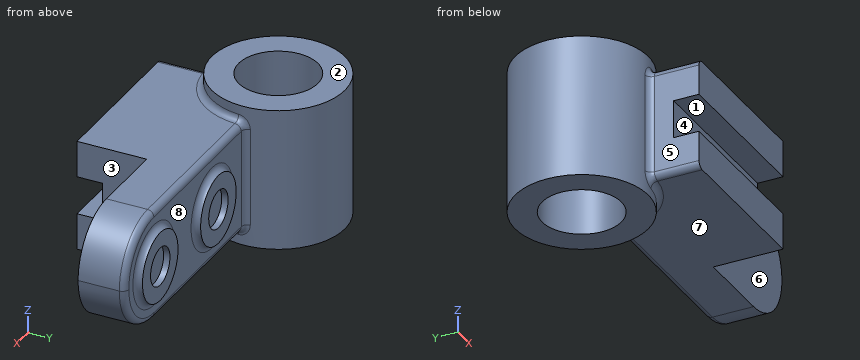
```python
from build123d import *

# Parameters (mm, degrees)
SKETCH3_R               = 21
SKETCH3_R_2             = 12.5
BOSS_EXTRUDE1_DEPTH     = 22.5
BOSS_EXTRUDE2_DEPTH     = 17.5
CUT_EXTRUDE1_DEPTH      = 85.877853413
CUT_EXTRUDE1_DEPTH_BACK = 53
BOSS_EXTRUDE3_DEPTH     = 2
CUT_EXTRUDE2_REACH      = 121.386
FILLET1_R               = 2


with BuildPart() as part:
    # Sketch3 → Boss-Extrude1 (new, symmetric)
    with BuildSketch(Plane.XY):
        with Locations(Location((0, 0, 0), (0, 0, 180))):
            Circle(SKETCH3_R)
        with Locations(Location((0, 0, 0), (0, 0, 180))):
            Circle(SKETCH3_R_2, mode=Mode.SUBTRACT)
    extrude(amount=BOSS_EXTRUDE1_DEPTH, both=True)

    # Sketch3<3> → Boss-Extrude2 (add, symmetric)
    with BuildSketch(Plane.XY):
        with BuildLine():
            ThreePointArc((21, 0), (14.849242405, -14.849242405), (0, -21))
            Line((0, -21), (0, -37))
            Line((0, -37), (52, -37))
            Line((52, -37), (52, -15))
            Line((52, -15), (111.255819071, -15))
            Line((111.255819071, -15), (111.255819071, 0))
            Line((111.255819071, 0), (21, 0))
        make_face()
    extrude(amount=BOSS_EXTRUDE2_DEPTH, both=True)

    # Sketch5 → Cut-Extrude1 (cut, two sides: drawn at the far end of the back side and taken through both)
    with BuildSketch(Plane(origin=(52, 0, 0), x_dir=(0, 0, -1), z_dir=(1, 0, 0)).offset(-CUT_EXTRUDE1_DEPTH_BACK)):
        Polygon((6, -176.247823966), (6, -37), (6, -29), (-6, -29), (-6, -37), (-6, -176.247823966), (-6, -454.743471899), (6, -454.743471899), align=None)
    extrude(amount=CUT_EXTRUDE1_DEPTH + CUT_EXTRUDE1_DEPTH_BACK, mode=Mode.SUBTRACT)

    # Sketch4 → Boss-Extrude3 (add)
    with BuildSketch(Plane(origin=(0, 0, 0), x_dir=(1, 0, 0), z_dir=(0, 1, 0))):
        with BuildLine():
            ThreePointArc((35, 0), (41, 6), (47, 0))
            Line((47, 0), (52, 0))
            ThreePointArc((52, 0), (41, 11), (30, 0))
            Line((30, 0), (35, 0))
        make_face()
        with BuildLine():
            Line((52, 0), (47, 0))
            ThreePointArc((47, 0), (41, -6), (35, 0))
            Line((35, 0), (30, 0))
            ThreePointArc((30, 0), (41, -11), (52, 0))
        make_face()
        with BuildLine():
            ThreePointArc((88, 0), (77, 11), (66, 0))
            Line((66, 0), (71, 0))
            ThreePointArc((71, 0), (77, 6), (83, 0))
            Line((83, 0), (88, 0))
        make_face()
        with BuildLine():
            Line((71, 0), (66, 0))
            ThreePointArc((66, 0), (77, -11), (88, 0))
            Line((88, 0), (83, 0))
            ThreePointArc((83, 0), (77, -6), (71, 0))
        make_face()
    extrude(amount=BOSS_EXTRUDE3_DEPTH)

    # Sketch4<3> → Cut-Extrude2 (cut, up to next)
    with BuildSketch(Plane(origin=(0, 0, 0), x_dir=(1, 0, 0), z_dir=(0, 1, 0)), mode=Mode.PRIVATE) as cut_extrude2_sk1:
        with BuildLine():
            ThreePointArc((77, 17.5), (89.374368671, 12.374368671), (94.5, 0))
            ThreePointArc((94.5, 0), (89.374368671, -12.374368671), (77, -17.5))
            Line((77, -17.5), (111.255819071, -17.5))
            Line((111.255819071, -17.5), (111.255819071, 17.5))
            Line((111.255819071, 17.5), (77, 17.5))
        make_face()
    cut_extrude2_tool1 = extrude(cut_extrude2_sk1.sketch, amount=-CUT_EXTRUDE2_REACH, mode=Mode.PRIVATE) & part.part
    add(cut_extrude2_tool1.solids().sort_by_distance((100.628245, 0, 0))[0], mode=Mode.SUBTRACT)

    # Fillet1
    fillet1_edges = [part.edges().sort_by_distance(p)[0] for p in [
        (14.849242405, -14.849242405, 17.5),
        (21, 0, 0),
        (0, -29, -17.5),
        (0, -21, 0),
        (0, -29, 17.5),
        (14.849242405, -14.849242405, -17.5),
        (66, 0, 0),
        (30, 0, 0),
        (49, 0, -17.5),
        (49, 0, 17.5),
        (94.5, 0, 0),
    ]]
    fillet(fillet1_edges, radius=FILLET1_R - 0.0001)  # a hair under: the kernel refuses the full size


solid = part.part
```
Geometry: final body of the model. Coordinates: model frame, mm. Face numbers are marked on the shaded views. A direction names the side the tool comes from. Coordinates: 2 decimals unless noted, no trailing zeros. Order: outer loops, then holes, each group sorted by start corner. A loop starts at its lowest first (then second) coordinate and runs counter-clockwise, first axis right, second up. Notation, with made-up numbers: (-25, -4.5) - (28, -4.5) arc R25 ccw to (28, 16.5) - close; hole circle Ø3 at (81.25, -35). An arc over 180 degrees is marked (long way). Return JSON: item names as keys, results as strings. Group by question number.
1. Cut plane B-B (y = 8.5). Output: boundary loops of the cut face in (x, z), plus the area to 3 significant figures.
2. Pin query (flat end, axial travel): pin 1 (6.5 mm diameter, centred on x = 40, z = -3, fed in from +Y); pin 2 (9.5 mm diameter, centred on x = 78, z = -0.5, fed in from +Y); pin 3 (1 mm diameter, centred on x = 29.5, y = -13, fed in from -Z). Return the tip coordinate at first contact, or that it passes through.
3. Material intervals for line 1 along Z through (x, y) = (11, -29.5); line 2 along Z through (x, y) = (57.5, -14); line 3 along Y through (x, z) = (48.5, 11.5), sorted ascending. Write a range as [from, to].
4. Pull-direction query (Z, two-part tool) for the marked faces 1, 2, 3 and 4; classes: pulls with the +Z half, pulls with the -Z half, needs draft (parallel to the pull), parting line crosses it, or undercut.
5. Set-up query: the marked faces 5, 6, 7 and 8. Return all of +Z, -Z, +X, -X, +Y, -Y with unobstructed straight access to the full face (end or side cutting, diameter ignored); none if empty.
Resolved:
{
 "1": {"outline": "(-19.2, -22.5) - (-9.17, -22.5) - (-9.17, 22.5) - (-19.2, 22.5) - close; (9.17, -22.5) - (19.2, -22.5) - (19.2, 22.5) - (9.17, 22.5) - close", "area": "903 mm²"},
 "2": {"pin 1": "stops at y = 2", "pin 2": "stops at y = 0", "pin 3": "stops at z = -17.5"},
 "3": {"line 1": "z = [-17.5, -6], [6, 17.5]", "line 2": "z = [-17.5, 17.5]", "line 3": "y = [-37, 0]"},
 "4": {"face 1": "undercut", "face 2": "pulls with the +Z half", "face 3": "needs draft", "face 4": "undercut"},
 "5": {"face 5": "+Z, -Z, -X, -Y", "face 6": "+Z, -Z, +X, -Y", "face 7": "-Z, +X, -Y", "face 8": "+Y"}
}
